Verification items for the finished model (mm, model axes). A direction names the side the tool comes from. Coordinates: 2 decimals unless noted, no trailing zeros. Order: outer loops, then holes, each group sorted by start corner. A loop starts at its lowest first (then second) coordinate and runs counter-clockwise, first axis right, second up.
Q1. Set-up check for faces 4 (the flat face through (-60, -28, 35)), 5 (the flat face through (67.5, 0, 19)): record each of +Z, -Z, +X, -X, +Y, -Y from which the full face is reachable in a straight line by a thin tool's end or side.
Q2. Cross-section at A-A, the plane z = 19.5. Record the boundary of the cut face in (x, y).
Q3. Cross-section at B-B, the plane x = -65. Record the boundary of the cut face in (y, z), and give its area (4 significant figures).
Q4. Thickness scan on line 1 (Y direction, x = -65, z = 2); line 2 (Y direction, x = 65, z = 0.95); line 3 (X direction, y = -32.5, z = 1.3). Record the ranges inside material, lowest first.
Q5. Draft check along X on faces 1 (the flat face through (-1, 37.5, 17)), 2 (the flat face through (-2, -35, 19)), 3 (the flat face through (-70, -2, 17)). Enter one of: pulls with the +X half, pulls with the -X half, needs draft (parallel to the pull), parting line crosses it, or undercut.
Q6. Depth check by flat-ended pin: P1, Ø8, axis at x = -54, y = 23.5, coming from the +Z side; P2, Ø12, axis at x = 25, y = -16, coming from the -Z side. Enter the tip coordinate at first touch or a pass-through.
Q7. Cross-section at C-C, the plane y = -27.5. Record the boundary of the cut face in (x, z).
Q8. Cross-section at D-D, the plane x = 60. Record the boundary of the cut face in (y, z).
from build123d import *

# Parameters (mm, degrees)
SKETCH1_W           = 140
SKETCH1_H           = 75
BOSS_EXTRUDE1_DEPTH = 35
SHELL1_T            = -2.5
SKETCH2_R           = 3
BOSS_EXTRUDE2_DEPTH = 32.5
SKETCH3_R           = 2.25
SKETCH3_R_2         = 2.5
CUT_EXTRUDE1_DEPTH  = 35
FILLET1_R           = 2


with BuildPart() as part:
    # Sketch1 → Boss-Extrude1 (new body)
    with BuildSketch(Plane.XY):
        Rectangle(SKETCH1_W, SKETCH1_H)
    extrude(amount=BOSS_EXTRUDE1_DEPTH)

    # Shell1
    shell1_openings = [part.faces().sort_by_distance(p)[0] for p in [
        (0, 0, 35),
    ]]
    offset(amount=SHELL1_T, openings=shell1_openings, kind=Kind.INTERSECTION)

    # Sketch2 → Boss-Extrude2 (add)
    with BuildSketch(Plane.XY.offset(2.5)):
        with Locations(Location((-60, -27.5, 0), (0, 0, 180))):
            Circle(SKETCH2_R)
        with Locations(Location((60, -27.5, 0), (0, 0, 180))):
            Circle(SKETCH2_R)
        with Locations(Location((-60, 27.5, 0), (0, 0, 180))):
            Circle(SKETCH2_R)
        with Locations(Location((60, 27.5, 0), (0, 0, 180))):
            Circle(SKETCH2_R)
    extrude(amount=BOSS_EXTRUDE2_DEPTH)

    # Sketch3 → Cut-Extrude1 (cut)
    with BuildSketch(Plane.XY):
        with Locations(Location((-65, -32.5, 0), (0, 0, 180))):
            Circle(SKETCH3_R)
        with Locations((65, -32.5)):
            Circle(SKETCH3_R_2)
        with Locations(Location((-65, 32.5, 0), (0, 0, 180))):
            Circle(SKETCH3_R)
        with Locations((65, 32.5)):
            Circle(SKETCH3_R_2)
    extrude(amount=CUT_EXTRUDE1_DEPTH, mode=Mode.SUBTRACT)

    # Fillet1
    fillet1_edges = [part.edges().sort_by_distance(p)[0] for p in [
        (-67.5, 0, 35),
        (70, -37.5, 17.5),
        (-70, 37.5, 17.5),
        (70, 37.5, 17.5),
    ]]
    fillet(fillet1_edges, radius=FILLET1_R)


solid = part.part
Check values:
1. face 4: +Z, +X, -X, +Y, -Y
1. face 5: +Z
2. outline: (-70, -37.5) - (68, -37.5) arc R2 ccw to (70, -35.5) - (70, 35.5) arc R2 ccw to (68, 37.5) - (-68, 37.5) arc R2 ccw to (-70, 35.5) - close; circle Ø6 at (-60, -27.5); circle Ø6 at (-60, 27.5); circle Ø6 at (60, -27.5); circle Ø6 at (60, 27.5); hole (-67.5, -35) - (67.5, -35) - (67.5, 35) - (-67.5, 35) - close
3. outline: (-37.5, 0) - (-34.75, 0) - (-34.75, 2.5) - (-35, 2.5) - (-35, 35) - (-37.5, 35) - close; (-30.25, 0) - (30.25, 0) - (30.25, 2.5) - (-30.25, 2.5) - close; (34.75, 0) - (37.5, 0) - (37.5, 35) - (35, 35) - (35, 2.5) - (34.75, 2.5) - close
3. area: 327.5 mm2
4. line 1: y = -37.5 to -34.75, -30.25 to 30.25, 34.75 to 37.5
4. line 2: y = -37.5 to -35, -30 to 30, 35 to 37.5
4. line 3: x = -70 to -67.25, -62.75 to 62.5, 67.5 to 70
5. face 1: needs draft
5. face 2: undercut
5. face 3: pulls with the -X half
6. P1: stops at z = 2.5
6. P2: stops at z = 0
7. outline: (-70, 0) - (70, 0) - (70, 35) - (67.5, 35) - (67.5, 2.5) - (63, 2.5) - (63, 35) - (57, 35) - (57, 2.5) - (-57, 2.5) - (-57, 35) - (-63, 35) - (-63, 2.5) - (-67.5, 2.5) - (-67.5, 33) arc R2 ccw to (-69.5, 35) - (-70, 35) - close
8. outline: (-37.5, 0) - (37.5, 0) - (37.5, 35) - (35, 35) - (35, 2.5) - (30.5, 2.5) - (30.5, 35) - (24.5, 35) - (24.5, 2.5) - (-24.5, 2.5) - (-24.5, 35) - (-30.5, 35) - (-30.5, 2.5) - (-35, 2.5) - (-35, 35) - (-37.5, 35) - close
